Drawing for the job (mm, zero at the part's lowest x, y, z). A direction names the side the tool comes from. Round coordinates to 2 decimals unless told otherwise and drop trailing zeros. Order: outer loops, then holes, each group sorted by start corner. A loop starts at its lowest first (then second) coordinate and runs counter-clockwise, first axis right, second up. Notation, with made-up numbers: (15, -16) - (65, -16) arc R22 cw to (65, 12) - close; hole circle Ø1 at (-35.75, 62.25). An arc over 180 degrees is marked (long way). Answer as a JSON object with one key per item and string values.
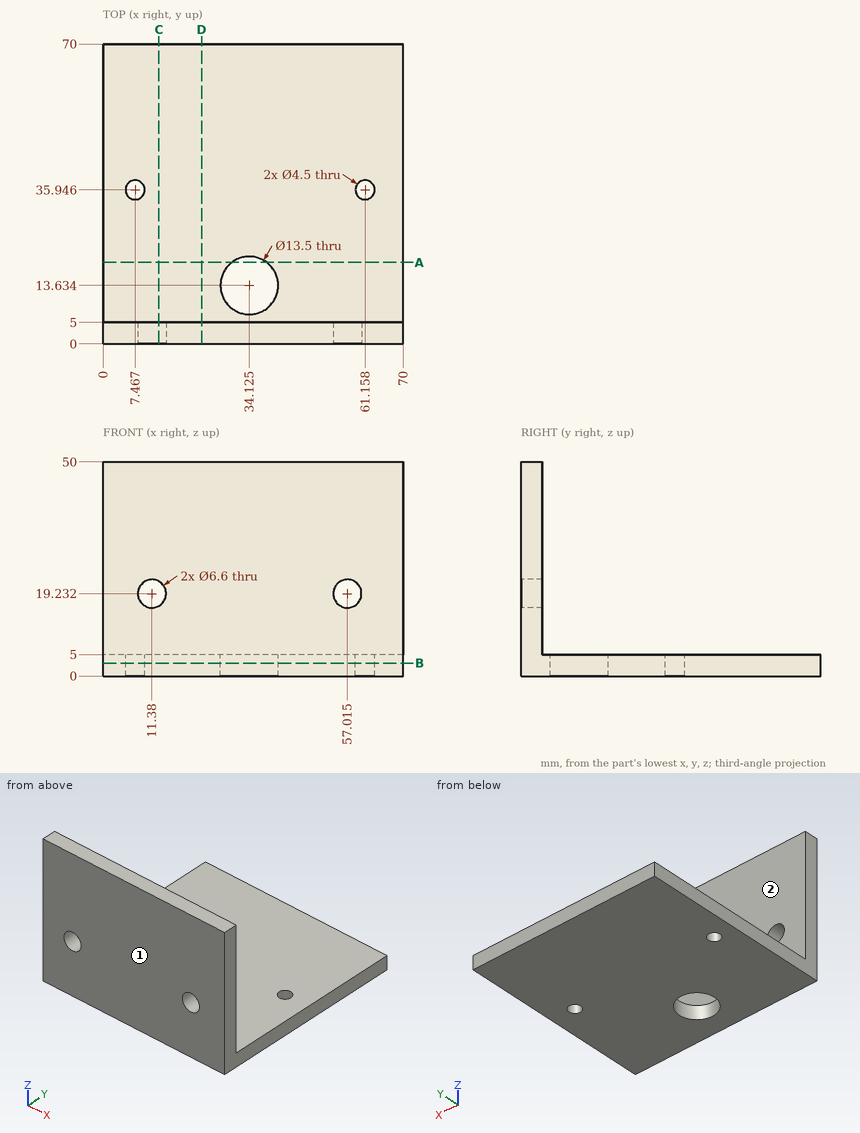
Item 1: Cut at B-B (z = 3). State how many separate pieces and enclosed holes the cut face has, plus the area to 4 significant figures.
Taken from the geometry:
{"separate pieces": "1", "enclosed holes": "3", "area": "4,725 mm2"}
Item 2: Cut at D-D (x = 23). Write the cut outline in (y, z).
Taken from the geometry:
{"outline": "(0, 0) - (70, 0) - (70, 5) - (5, 5) - (5, 50) - (0, 50) - close"}
Item 3: Cut at A-A (y = 19). Write the cut outline in (x, z).
Taken from the geometry:
{"outline": "(0, 0) - (30.03, 0) - (30.03, 5) - (0, 5) - close; (38.22, 0) - (70, 0) - (70, 5) - (38.22, 5) - close"}
Item 4: Probe L1, parallel to Z at x = 9.5, y = 41; L2, parallel to Z at x = 13, y = 3.5 (1 decimal). List the from-to ranges inside material, lowest first. Write a range as from..to.
Taken from the geometry:
{"L1": "0..5", "L2": "0..16.4, 22.1..50"}
Item 5: Tool access for the marked faces 1 and 2: list every direction of +Z, -Z, +X, -X, +Y, -Y with a clear straight run to the whole face (end or side of a thin tool).
Taken from the geometry:
{"face 1": "+Z, -Z, +X, -X, -Y", "face 2": "+Z, +X, -X, +Y"}
Item 6: Drop flat-ended pins along their axis: P1, Ø12, axis at x = 27, y = 52, coming from the +Z side; P2, Ø13.5, axis at x = 43.5, z = 37.5, coming from the +Y side; P3, Ø12, axis at x = 34.12, y = 13.63, coming from the +Z side. Give the stop position or say it passes through.
Taken from the geometry:
{"P1": "z = 5", "P2": "y = 5", "P3": "through"}
Item 7: Cut at C-C (x = 13). Write the cut outline in (y, z).
Taken from the geometry:
{"outline": "(0, 0) - (70, 0) - (70, 5) - (5, 5) - (5, 16.36) - (0, 16.36) - close; (0, 22.11) - (5, 22.11) - (5, 50) - (0, 50) - close"}
